Geometry: final body of the model. Coordinates: model frame, mm. A direction names the side the tool comes from. Give positions to 0.01 mm unless a question says otherwise; leave off trailing zeros. Write each loop counter-clockwise with the first axis right and the second up, starting at its lowest first coordinate (ties: lowest second). Pieces come first, ordered by that corner, then holes. Notation, with made-up numbers: M -28,87.5 L -20,87.5 A7 cw -20,100.5 Z; hole C 62,35.5 d4. An arc over 180 degrees is marked long. Use one line per item in the form item = value. Start each with the question number.
Item 1: Contact query for a flat-ended pin moving along its axis: P1, Ø1.5, axis at x = 0, y = -9.5, coming from the +Z side. Output: stop coordinate, or through.
Item 2: Material intervals for line 1 along Y through (x, z) = (-0.7, -1.6); line 2 along Y through (x, z) = (1.5, -1); line 3 along Z through (x, y) = (-0.7, -2.5), sorted ascending. Write a range as from..to.
Item 3: Section query B-B on x = 0. Return loops of the section in (y, z), then the cut area to 3 significant figures.
Item 4: Section query A-A on z = 0. Return loops of the section in (x, y).
Item 5: Access query for faces 1 (the cylindrical face through (1.736, -3.735, 0.385)), 2 (the cylindrical face through (-1.26, -30.14, 0.17)), 3 (the flat face through (0, -33.274, 0)). Directions: +Z, -Z, +X, -X, +Y, -Y. A direction counts if a zero-diameter tool reaches every point of the face in a straight line with its end or side. Return the directions, or none.
Item 6: Section query C-C on y = -19.5. Return loops of the section in (x, z), then the cut area to 3 significant figures.
from build123d import *

# Parameters (mm, degrees)
SKETCH1_W = 0.254
SKETCH1_H = 0.254


with BuildPart() as part:
    # Sketch1 → Revolve2 (revolve)
    with BuildSketch(Plane.XY, mode=Mode.PRIVATE) as revolve2_sk:
        Polygon((0, -33.274), (0, 0), (1.778, 0), (1.778, -26.924), (1.27, -26.924), (1.27, -33.274), align=None)
        with Locations((1.905, -7.493)):
            Rectangle(SKETCH1_W, SKETCH1_H)
    revolve(revolve2_sk.sketch.rotate(Axis((0, 0, 0), (0, 1, 0)), 90), axis=Axis((0, 0, 0), (0, 1, 0)))


solid = part.part
Answer sheet:
q1.P1 = 1.78
q2.line_1 = -26.92..0
q2.line_2 = -7.62..-7.37
q2.line_3 = -1.63..1.63
q3.outline = M -33.27,-1.27 L -26.92,-1.27 L -26.92,-1.78 L -7.62,-1.78 L -7.62,-2.03 L -7.37,-2.03 L -7.37,-1.78 L 0,-1.78 L 0,1.78 L -7.37,1.78 L -7.37,2.03 L -7.62,2.03 L -7.62,1.78 L -26.92,1.78 L -26.92,1.27 L -33.27,1.27 Z
q3.area = 112 mm2
q4.outline = M -2.03,-7.62 L -1.78,-7.62 L -1.78,-26.92 L -1.27,-26.92 L -1.27,-33.27 L 1.27,-33.27 L 1.27,-26.92 L 1.78,-26.92 L 1.78,-7.62 L 2.03,-7.62 L 2.03,-7.37 L 1.78,-7.37 L 1.78,0 L -1.78,0 L -1.78,-7.37 L -2.03,-7.37 Z
q5.face_1 = +Y
q5.face_2 = -Y
q5.face_3 = +Z, -Z, +X, -X, -Y
q6.outline = C 0,0 d3.56
q6.area = 9.93 mm2
